```python
from build123d import *

# Parameters (mm, degrees)
CROQUIS1_W                   = 85
CROQUIS1_H                   = 45
SALIENTE_EXTRUIR1_DEPTH      = 45
SALIENTE_EXTRUIR2_DEPTH      = 25
SALIENTE_EXTRUIR2_DEPTH_BACK = 108
CROQUIS2_R                   = 20
CROQUIS7_R                   = 19.05
SALIENTE_EXTRUIR3_DEPTH      = 25
CROQUIS10_R                  = 16.961855078
CORTAR_EXTRUIR2_DEPTH        = 45
CROQUIS12_R                  = 19.05
CORTAR_EXTRUIR3_DEPTH        = 159


with BuildPart() as part:
    # Croquis1 → Saliente-Extruir1 (new body)
    with BuildSketch(Plane.XY):
        Rectangle(CROQUIS1_W, CROQUIS1_H)
    extrude(amount=SALIENTE_EXTRUIR1_DEPTH)

    # Croquis2 → Saliente-Extruir2 (add, two sides: drawn at the far end of the back side and taken through both)
    with BuildSketch(Plane(origin=(42.5, 0, 0), x_dir=(0, 0, -1), z_dir=(1, 0, 0)).offset(-SALIENTE_EXTRUIR2_DEPTH_BACK)):
        with Locations((-22.5, 0)):
            Circle(CROQUIS2_R)
    extrude(amount=SALIENTE_EXTRUIR2_DEPTH + SALIENTE_EXTRUIR2_DEPTH_BACK)

    # Croquis7 → Saliente-Extruir3 (add)
    with BuildSketch(Plane.XZ.offset(22.5)):
        with Locations(Location((0, 22.39581729, 0), (0, 0, 180))):
            Circle(CROQUIS7_R)
    extrude(amount=SALIENTE_EXTRUIR3_DEPTH)

    # Croquis10 → Cortar-Extruir2 (cut)
    with BuildSketch(Plane(origin=(0, -47.5, 0), x_dir=(-1, 0, 0), z_dir=(0, -1, 0))):
        with Locations(Location((0, -22.64581729, 0), (0, 0, 180))):
            Circle(CROQUIS10_R)
    extrude(amount=-CORTAR_EXTRUIR2_DEPTH, mode=Mode.SUBTRACT)

    # Croquis12 → Cortar-Extruir3 (cut)
    with BuildSketch(Plane(origin=(67.5, 0, 0), x_dir=(0, 0, -1), z_dir=(1, 0, 0))):
        with Locations((-22.75, 0)):
            Circle(CROQUIS12_R)
    extrude(amount=-CORTAR_EXTRUIR3_DEPTH, mode=Mode.SUBTRACT)


solid = part.part
```
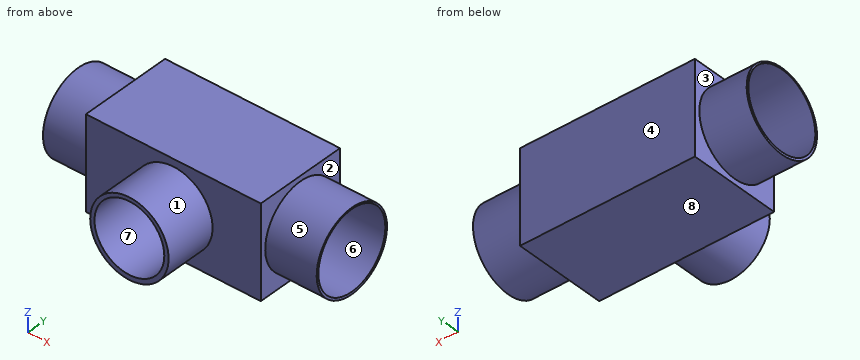
CAD build for the part. Positions are in the model's coordinates, mm. Face numbers are marked on the shaded views. A direction names the side the tool comes from. Coordinates: 2 decimals unless noted, no trailing zeros. Write each loop counter-clockwise with the first axis right and the second up, starting at its lowest first coordinate (ties: lowest second). Pieces come first, ordered by that corner, then holes.
(1) Drill centre lines: probe 1 along Y at (x, z) = (28, 22.75); probe 2 along Z at (x, y) = (0, -17); probe 3 along Z at (x, y) = (0, -37). Where is each one in solid material? Low to high.
(2) Cut at D-D, the plane x = 2. List the corners of the cut face in (y, z).
(3) Cut at A-A, the plane y = -7. List the corners of the cut face in (x, z) (3 decimals).
(4) Two-plate mould, pull along Z, no slides. Class the marked faces 5, 6, 7 and 8: +Z half, -Z half, draft (parallel to the pull), parting line (faces both ways), or undercut.
(5) Cut at B-B, the plane x = -35.5. List the corners of the cut face in (y, z), and give its area (3 significant figures).
(6) 3-axis set-ups, long thin cutter, end or side, ignore diameter. For the marked faces 1, 2, 3 and 4: which of +Z, -Z, +X, -X, +Y, -Y reach the whole face in a straight line?
(7) Flat gauge pins, fed straight in: pin 1 (20.5 mm diameter, centred on x = 0, z = 22.65, fed in from -Y); pin 2 (13.5 mm diameter, centred on x = 21, z = 30.5, fed in from -Y); pin 3 (1 mm diameter, centred on x = -8, y = -33, fed in from +Z); pin 4 (1 mm diameter, centred on x = -3.5, z = 9, fed in from -Y). Where does each tip first touch, or does it go through?
(8) Cut at C-C, the plane z = 34.5. List the corners of the cut face in (x, y).
Geometry says:
1. probe 1: y = -22.5 to -19.05, 19.05 to 22.5
1. probe 2: z = 0 to 5.68, 39.61 to 45
1. probe 3: z = 3.35 to 5.68, 39.61 to 41.45
2. outline: (-47.5, 3.45) - (-22.5, 3.45) - (-22.5, 0) - (22.5, 0) - (22.5, 45) - (-22.5, 45) - (-22.5, 41.34) - (-47.5, 41.34) - (-47.5, 39.49) - (-9.09, 39.49) arc R19.05 cw (long way) to (-8.7, 5.8) - (-47.5, 5.8) - close
3. outline: (-65.5, 3.765) - (-42.5, 3.765) - (-42.5, 0) - (42.5, 0) - (42.5, 3.765) - (67.5, 3.765) - (67.5, 5.033) - (-65.5, 5.033) - close; (-65.5, 40.467) - (67.5, 40.467) - (67.5, 41.235) - (42.5, 41.235) - (42.5, 45) - (-42.5, 45) - (-42.5, 41.235) - (-65.5, 41.235) - close
4. face 5: parting line
4. face 6: undercut
4. face 7: undercut
4. face 8: -Z half
5. outline: (-22.5, 0) - (22.5, 0) - (22.5, 45) - (-22.5, 45) - close; hole circle Ø38.1 at (0, 22.75)
5. area: 885 mm2
6. face 1: -Y
6. face 2: +X
6. face 3: -X
6. face 4: +Z, -Z, +X, -X, +Y
7. pin 1: stops at y = 15.99
7. pin 2: stops at y = -47.5
7. pin 3: stops at z = 39.91
7. pin 4: stops at y = 12.64
8. outline: (-65.5, -16) - (-42.5, -16) - (-42.5, -22.5) - (-14.71, -22.5) - (-14.71, -47.5) - (-12.13, -47.5) - (-12.13, -14.99) - (-65.5, -14.99) - close; (-65.5, 14.99) - (67.5, 14.99) - (67.5, 16) - (42.5, 16) - (42.5, 22.5) - (-42.5, 22.5) - (-42.5, 16) - (-65.5, 16) - close; (12.13, -47.5) - (14.71, -47.5) - (14.71, -22.5) - (42.5, -22.5) - (42.5, -16) - (67.5, -16) - (67.5, -14.99) - (12.13, -14.99) - close
